Autodesk Inventor part; units mm, degrees
ref_plane "YZ Plane" through (0, 0, 0) normal (1, 0, 0) x (0, 1, 0)
ref_plane "XZ Plane" through (0, 0, 0) normal (0, 1, 0) x (-1, 0, 0)
ref_plane "XY Plane" through (0, 0, 0) normal (0, 0, 1) x (1, 0, 0)
sketch "Sketch1" plane through (0, 0, 0) normal (0, 0, 1) x (1, 0, 0)
  line L0 (0, 0) -> (0, 50) construction
  line L1 (0, 50) -> (30, 50) construction
  line L2 (30, 50) -> (30, 15)
  line L3 (30, 15) -> (90, 15)
  line L4 (90, 15) -> (90, 50)
  line L5 (90, 50) -> (85, 50)
  line L6 (85, 50) -> (85, 20)
  line L7 (85, 20) -> (35, 20)
  line L8 (35, 20) -> (35, 50)
  line L9 (35, 50) -> (30, 50)
  dimension "d0" = 50
  dimension "d1" = 30
  dimension "d2" = 35
  dimension "d3" = 60
  dimension "d4" = 35
  dimension "d5" = 5
  dimension "d6" = 30
  dimension "d7" = 50
revolve "Revolution1" add sketch "Sketch1" angle 60 about axis through (0, 0, 0) along (0, 1, 0)
properties part number "track z2201"
Work out the finished part from the listing and answer in its coordinate system (mm). A direction names the side the tool comes from. Round coordinates to 2 decimals unless told otherwise and drop trailing zeros. Loops run counter-clockwise (first coordinate to the right, second up) from the corner with the lowest first, then second, coordinate; pieces in that order, holes last. Notation, with made-up numbers: (24, 40.25) -> (76, 40.25) arc R21 ccw to (76, 76.25) -> close; hole circle Ø7 at (-13.5, 13). An arc over 180 degrees is marked (long way). Use one line per item in the form item = value.
(1) Find section C-C on x = 82.5. Give the vertices of the cut face in (y, z), then the cut area to 3 significant figures.
Answer list:
outline = (15, -35.97) -> (50, -35.97) -> (50, -20.46) -> (20, -20.46) -> (20, 0) -> (15, 0) -> close
area = 645 mm2
(2) A tool of negligible diameter and unlimited length cuts with its end or side. For faces 1 (the cylindrical face through (30.438, 35.21, -17.277)), 2 (the cylindrical face through (73.3, 34.79, -43.04)), 3 (the flat face through (27, 50, -15)), from which of +Z, -Z, +X, -X, +Y, -Y can it reach the whole face along a straight path? Write none if from no direction.
Answer list:
face_1 = -Z, +Y
face_2 = +Z, +Y
face_3 = +Z, -Z, +X, -X, +Y
(3) Find section D-D on z = -45.5. Give the vertices of the cut face in (x, y), then the cut area to 3 significant figures.
Answer list:
outline = (26.27, 15) -> (77.65, 15) -> (77.65, 50) -> (71.8, 50) -> (71.8, 20) -> (26.27, 20) -> close
area = 433 mm2
(4) Straight lines are drawn through the part: line 1 (Y direction, x = 27.5, z = -25.5); line 2 (X direction, y = 42.5, z = -14); line 3 (X direction, y = 43.5, z = -24). For each, find the intervals that lie inside material, in ascending order.
Answer list:
line_1 = 15 to 20
line_2 = 26.53 to 32.08, 83.84 to 88.9
line_3 = 18 to 25.48, 81.54 to 86.74
(5) For a pull along X with two mould halves and no side action, classify faces 4 (the flat face through (62.1, 19.6, 0)), 5 (the cylindrical face through (78.27, 32.75, -44.43)), 6 (the flat face through (51, 20, -29)) as released by +X, released by -X, zero draft, split by the parting line, or undercut.
Answer list:
face_4 = zero draft
face_5 = released by +X
face_6 = undercut
(6) Find section A-A on y = 40. Give the vertices of the cut face in (x, z), then the cut area to 3 significant figures.
Answer list:
outline = (15, -25.98) -> (17.5, -30.31) arc R35 ccw to (35, 0) -> (30, 0) arc R30 cw to start; (42.5, -73.61) -> (45, -77.94) arc R90 ccw to (90, 0) -> (85, 0) arc R85 cw to start
area = 628 mm2
(7) Flat-ended cylindrical pins translate along their axes: P1, Ø6, axis at y = 25, z = -56.5, coming from the +X side; P2, Ø10, axis at y = 37.5, z = -57, coming from the -X side; P3, Ø4, axis at y = 25.5, z = -31.5, coming from the +X side. Find the tip coordinate at first contact, or state that the pin passes through.
Answer list:
P1 = 72.37
P2 = 58.15
P3 = 85.03
(8) Find section B-B on z = -13. Give the vertices of the cut face in (x, y), then the cut area to 3 significant figures.
Answer list:
outline = (27.04, 15) -> (89.06, 15) -> (89.06, 50) -> (84, 50) -> (84, 20) -> (32.5, 20) -> (32.5, 50) -> (27.04, 50) -> close
area = 626 mm2
